```python
from build123d import *

# Parameters (mm, degrees)
SKETCH_1_W          = 20
SKETCH_1_H          = 20
EXTRUDE_2_DEPTH     = 500
CUT_EXTRUDE_1_REACH = 502.5
SKETCH_2_R          = 2.55
SKETCH_3_W          = 20
SKETCH_3_H          = 50
EXTRUDE_3_DEPTH     = 20
SKETCH_4_R          = 2.55
CUT_EXTRUDE_2_DEPTH = 20
SKETCH_5_W          = 20
SKETCH_5_H          = 20
CUT_EXTRUDE_3_DEPTH = 250
CUT_EXTRUDE_4_REACH = 503.298
SKETCH_6_R          = 2.55


with BuildPart() as part:
    # 草图1 → 凸台-拉伸2 (new body)
    with BuildSketch(Plane.XY):
        Rectangle(SKETCH_1_W, SKETCH_1_H)
    extrude_2 = extrude(amount=EXTRUDE_2_DEPTH)

    # 草图2 → 切除-拉伸1 (cut, up to next)
    with BuildSketch(Plane(origin=(10, 0, 0), x_dir=(0, 0, -1), z_dir=(1, 0, 0)), mode=Mode.PRIVATE) as cut_extrude_1_sk1:
        with Locations((-10, 0)):
            Circle(SKETCH_2_R)
    cut_extrude_1_tool1 = extrude(cut_extrude_1_sk1.sketch, amount=-CUT_EXTRUDE_1_REACH, mode=Mode.PRIVATE) & part.part
    # 草图2 → 切除-拉伸1 (cut, up to next)
    with BuildSketch(Plane(origin=(10, 0, 0), x_dir=(0, 0, -1), z_dir=(1, 0, 0)), mode=Mode.PRIVATE) as cut_extrude_1_sk2:
        with Locations((-40, 0)):
            Circle(SKETCH_2_R)
    cut_extrude_1_tool2 = extrude(cut_extrude_1_sk2.sketch, amount=-CUT_EXTRUDE_1_REACH, mode=Mode.PRIVATE) & part.part
    add(cut_extrude_1_tool1.solids().sort_by_distance((10, 0, 10))[0], mode=Mode.SUBTRACT)
    add(cut_extrude_1_tool2.solids().sort_by_distance((10, 0, 40))[0], mode=Mode.SUBTRACT)

    # 草图3 → 凸台-拉伸3 (add)
    with BuildSketch(Plane.XZ.offset(10)):
        with Locations((0, 25)):
            Rectangle(SKETCH_3_W, SKETCH_3_H)
    extrude_3 = extrude(amount=EXTRUDE_3_DEPTH)

    # 草图4 → 切除-拉伸2 (cut)
    with BuildSketch(Plane(origin=(10, 0, 0), x_dir=(0, 0, -1), z_dir=(1, 0, 0))):
        with Locations((-40, -20)):
            Circle(SKETCH_4_R)
        with Locations((-10, -20)):
            Circle(SKETCH_4_R)
    extrude(amount=-CUT_EXTRUDE_2_DEPTH, mode=Mode.SUBTRACT)

    # 草图5 → 切除-拉伸3 (cut)
    with BuildSketch(Plane.XY.offset(500)):
        Rectangle(SKETCH_5_W, SKETCH_5_H)
    extrude(amount=-CUT_EXTRUDE_3_DEPTH, mode=Mode.SUBTRACT)

    # 镜向2: 凸台-拉伸2, 凸台-拉伸3 across plane
    add(extrude_2.mirror(Plane(origin=(0, 0, 250), x_dir=(1, 0, 0), z_dir=(0, 0, -1))))
    add(extrude_3.mirror(Plane(origin=(0, 0, 250), x_dir=(1, 0, 0), z_dir=(0, 0, -1))))

    # 草图6 → 切除-拉伸4 (cut, up to next)
    with BuildSketch(Plane(origin=(10, 0, 0), x_dir=(0, 0, -1), z_dir=(1, 0, 0)), mode=Mode.PRIVATE) as cut_extrude_4_sk1:
        with Locations((-490, 0)):
            Circle(SKETCH_6_R)
    cut_extrude_4_tool1 = extrude(cut_extrude_4_sk1.sketch, amount=-CUT_EXTRUDE_4_REACH, mode=Mode.PRIVATE) & part.part
    # 草图6 → 切除-拉伸4 (cut, up to next)
    with BuildSketch(Plane(origin=(10, 0, 0), x_dir=(0, 0, -1), z_dir=(1, 0, 0)), mode=Mode.PRIVATE) as cut_extrude_4_sk2:
        with Locations((-460, 0)):
            Circle(SKETCH_6_R)
    cut_extrude_4_tool2 = extrude(cut_extrude_4_sk2.sketch, amount=-CUT_EXTRUDE_4_REACH, mode=Mode.PRIVATE) & part.part
    # 草图6 → 切除-拉伸4 (cut, up to next)
    with BuildSketch(Plane(origin=(10, 0, 0), x_dir=(0, 0, -1), z_dir=(1, 0, 0)), mode=Mode.PRIVATE) as cut_extrude_4_sk3:
        with Locations((-460, -20)):
            Circle(SKETCH_6_R)
    cut_extrude_4_tool3 = extrude(cut_extrude_4_sk3.sketch, amount=-CUT_EXTRUDE_4_REACH, mode=Mode.PRIVATE) & part.part
    # 草图6 → 切除-拉伸4 (cut, up to next)
    with BuildSketch(Plane(origin=(10, 0, 0), x_dir=(0, 0, -1), z_dir=(1, 0, 0)), mode=Mode.PRIVATE) as cut_extrude_4_sk4:
        with Locations((-490, -20)):
            Circle(SKETCH_6_R)
    cut_extrude_4_tool4 = extrude(cut_extrude_4_sk4.sketch, amount=-CUT_EXTRUDE_4_REACH, mode=Mode.PRIVATE) & part.part
    # 草图6 → 切除-拉伸4 (cut, up to next)
    with BuildSketch(Plane(origin=(10, 0, 0), x_dir=(0, 0, -1), z_dir=(1, 0, 0)), mode=Mode.PRIVATE) as cut_extrude_4_sk5:
        with Locations((-10, 0)):
            Circle(SKETCH_6_R)
    cut_extrude_4_tool5 = extrude(cut_extrude_4_sk5.sketch, amount=-CUT_EXTRUDE_4_REACH, mode=Mode.PRIVATE) & part.part
    # 草图6 → 切除-拉伸4 (cut, up to next)
    with BuildSketch(Plane(origin=(10, 0, 0), x_dir=(0, 0, -1), z_dir=(1, 0, 0)), mode=Mode.PRIVATE) as cut_extrude_4_sk6:
        with Locations((-40, 0)):
            Circle(SKETCH_6_R)
    cut_extrude_4_tool6 = extrude(cut_extrude_4_sk6.sketch, amount=-CUT_EXTRUDE_4_REACH, mode=Mode.PRIVATE) & part.part
    add(cut_extrude_4_tool1.solids().sort_by_distance((10, 0, 490))[0], mode=Mode.SUBTRACT)
    add(cut_extrude_4_tool2.solids().sort_by_distance((10, 0, 460))[0], mode=Mode.SUBTRACT)
    add(cut_extrude_4_tool3.solids().sort_by_distance((10, -20, 460))[0], mode=Mode.SUBTRACT)
    add(cut_extrude_4_tool4.solids().sort_by_distance((10, -20, 490))[0], mode=Mode.SUBTRACT)
    add(cut_extrude_4_tool5.solids().sort_by_distance((10, 0, 10))[0], mode=Mode.SUBTRACT)
    add(cut_extrude_4_tool6.solids().sort_by_distance((10, 0, 40))[0], mode=Mode.SUBTRACT)


solid = part.part
```
Work out the finished part from the listing and answer in its coordinate system (mm). A direction names the side the tool comes from. Coordinates: 2 decimals unless noted, no trailing zeros. Write each loop counter-clockwise with the first axis right and the second up, starting at its lowest first coordinate (ties: lowest second). Pieces come first, ordered by that corner, then holes.
Q1. Each of these flat-tipped pins is pushed along its axis until it touches: pin 1 Ø10 at (x, z) = (0, 164.5) entering from -Y; pin 2 Ø4 at (y, z) = (-20, 460) entering from +X. Where does it stop, or does it pass through?
Q2. Find the intervals of material crossed by line 1 (Z direction, x = 8, y = -27); line 2 (Z direction, x = 0, y = -21.5); line 3 (Z direction, x = -5.75, y = -2), in increasing order.
Q3. A cutting plane is placed at B-B, the plane z = 278. Give the vertices of the cut face in (x, y).
Q4. Determine the mould class of faces 1 (the face through (0, -20, 50)), 2 (the face through (0, -10, 0)), 3 (the face through (0, -30, 475)) for opening direction Z: released by +Z, released by -Z, zero draft, split by the parting line, or undercut.
Q5. Which of the six approach directions +Z, -Z, +X, -X, +Y, -Y give full straight-line access (tool end or side, diameter ignored) to faces 4 (the face through (0, -10, 500)), 5 (the face through (0, -10, 253))?
Q6. A cutting plane is placed at A-A, the plane x = 3. State how many separate pieces and enclosed holes the cut face has, then the cut area to 3 significant figures.
Findings below:
1. pin 1: stops at y = -10
1. pin 2: passes through
2. line 1: z = 0 to 50, 450 to 500
2. line 2: z = 0 to 7.94, 12.06 to 37.94, 42.06 to 50, 450 to 457.94, 462.06 to 487.94, 492.06 to 500
2. line 3: z = 0 to 8.42, 11.58 to 38.42, 41.58 to 458.42, 461.58 to 488.42, 491.58 to 500
3. outline: (-10, -10) - (10, -10) - (10, 10) - (-10, 10) - close
4. face 1: undercut
4. face 2: released by -Z
4. face 3: zero draft
5. face 4: +Z, +X, -X, +Y, -Y
5. face 5: +X, -X, -Y
6. separate pieces: 1
6. enclosed holes: 8
6. area: 11,800 mm2
